from build123d import *

# Parameters (mm, degrees)
SKETCH_1_R          = 4
EXTRUDE_1_DEPTH     = 5
SKETCH_2_R          = 2.5
EXTRUDE_2_DEPTH     = 10
CHAMFER_1_SIZE      = 0.5
CUT_EXTRUDE_1_DEPTH = 4
FILLET_1_R          = 1
FILLET_2_R          = 0.5


with BuildPart() as part:
    # Эскиз1 → Вытянуть1 (new body)
    with BuildSketch(Plane(origin=(0, 0, 0), x_dir=(0, 0, -1), z_dir=(1, 0, 0))):
        Circle(SKETCH_1_R)
    extrude(amount=EXTRUDE_1_DEPTH)

    # Эскиз2 → Вытянуть2 (add)
    with BuildSketch(Plane(origin=(5, 0, 0), x_dir=(0, 0, -1), z_dir=(1, 0, 0))):
        Circle(SKETCH_2_R)
    extrude(amount=EXTRUDE_2_DEPTH)

    # Фаска1
    chamfer_1_edges = [part.edges().sort_by_distance(p)[0] for p in [
        (15, 0, 2.5),
    ]]
    chamfer(chamfer_1_edges, length=CHAMFER_1_SIZE)

    # Эскиз3 → Вырез-Вытянуть1 (cut)
    with BuildSketch(Plane.ZY):
        Polygon((0, 2.309401077), (-2, 1.154700538), (-2, -1.154700538), (0, -2.309401077), (2, -1.154700538), (2, 1.154700538), align=None)
    extrude(amount=-CUT_EXTRUDE_1_DEPTH, mode=Mode.SUBTRACT)

    # Скругление1
    fillet_1_edges = [part.edges().sort_by_distance(p)[0] for p in [
        (4, 1.732050808, 1),
        (4, 0, 2),
        (4, -1.732050808, 1),
        (4, -1.732050808, -1),
        (4, 0, -2),
        (4, 1.732050808, -1),
    ]]
    fillet(fillet_1_edges, radius=FILLET_1_R)

    # Скругление2
    fillet_2_edges = [part.edges().sort_by_distance(p)[0] for p in [
        (0, 0, 4),
    ]]
    fillet(fillet_2_edges, radius=FILLET_2_R)


solid = part.part
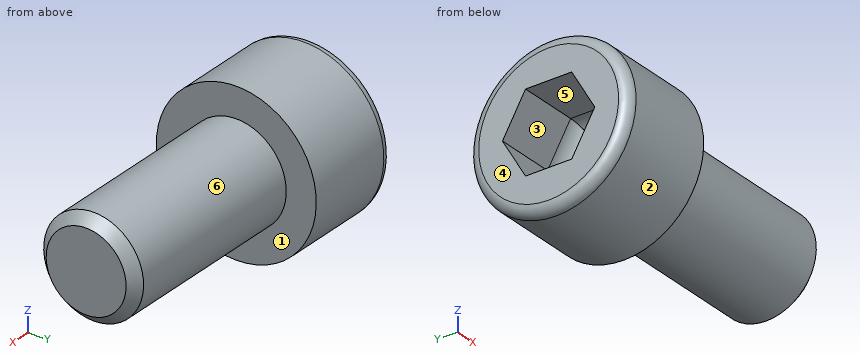
Can you work these out from the model? Positions are in its coordinate system, mm. Face numbers are marked on the shaded views. A direction names the side the tool comes from. Round coordinates to 2 decimals unless told otherwise and drop trailing zeros. Order: outer loops, then holes, each group sorted by start corner. A loop starts at its lowest first (then second) coordinate and runs counter-clockwise, first axis right, second up. Notation, with made-up numbers: (19.5, 73.5) -> (45.5, 73.5) arc R16 ccw to (45.5, 102.5) -> close; hole circle Ø1 at (56.25, 7.25). An arc over 180 degrees is marked (long way). Write each question's results on one line, items separated by ' | '. Start each with the question number.
Item 1: Please list where these lines run through material, in increasing order: L1, parallel to X at y = -1.25, z = 2.75; L2, parallel to Z at x = 2.75, y = 1; L3, parallel to Z at x = 3, y = 1.25.
Item 2: If we section it at A-A, the plane x = 2.5: Write out the boundary of the cut face in (y, z).
Item 3: If we section it at B-B, the plane y = 0: Write out the boundary of the cut face in (x, z), then the cut area to 3 significant figures.
Item 4: Thinking about a two-plate mould opening in Y: for the marked faces 1, 2 and 3, which applies, +Y half, -Y half, draft (parallel to the pull), parting line (faces both ways), or undercut?
Item 5: Will these pins go through, and if not, where does the flat tip stop? pin 1 (1 mm diameter, centred on x = 6.5, y = 2.5, fed in from -Z); pin 2 (0.6 mm diameter, centred on y = 0, z = -0.5, fed in from -X); pin 3 (1.5 mm diameter, centred on x = 7, z = -3, fed in from -Y); pin 4 (4 mm diameter, centred on y = 2, z = -0.5, fed in from +X).
Item 6: Which directions (+Z, -Z, +X, -X, +Y, -Y) give clear straight access to the entire face, cutting with the end or side of a thin tool? Please do the marked faces 4, 5 and 6.
Item 7: If we section it at C-C, the plane x = 6.25: Write out the boundary of the cut face in (y, z).
Results:
1) L1: x = 0 to 5 | L2: z = -3.87 to -2, 2 to 3.87 | L3: z = -3.8 to -1.83, 1.83 to 3.8
2) outline: circle Ø8 at (0, 0); hole (-2.31, 0) -> (-1.15, -2) -> (1.15, -2) -> (2.31, 0) -> (1.15, 2) -> (-1.15, 2) -> close
3) outline: (0, -3.5) arc R0.5 ccw to (0.5, -4) -> (5, -4) -> (5, -2.5) -> (14.5, -2.5) -> (15, -2) -> (15, 2) -> (14.5, 2.5) -> (5, 2.5) -> (5, 4) -> (0.5, 4) arc R0.5 ccw to (0, 3.5) -> (0, 2) -> (3, 2) arc R1 cw to (4, 1) -> (4, -1) arc R1 cw to (3, -2) -> (0, -2) -> close | area: 74.1 mm2
4) face 1: draft | face 2: parting line | face 3: undercut
5) pin 1: stops at z = -1.5 | pin 2: stops at x = 4 | pin 3: stops at y = -1.09 | pin 4: stops at x = 15
6) face 4: +Z, -Z, -X, +Y, -Y | face 5: -X | face 6: +X
7) outline: circle Ø5 at (0, 0)
